For this review, take the finished solid that the model builds, in its own axes (mm). Face numbers are marked on the shaded views. A direction names the side the tool comes from. Coordinates: 2 decimals unless noted, no trailing zeros. Order: outer loops, then holes, each group sorted by start corner. A loop starts at its lowest first (then second) coordinate and runs counter-clockwise, first axis right, second up. Notation, with made-up numbers: M -1.5,-18 L 47.5,-18 A9 ccw 47.5,-9 Z; hole C -34.75,-33.75 d4. An arc over 180 degrees is marked long. Use CSV: the item, a comma, the result in double quotes.
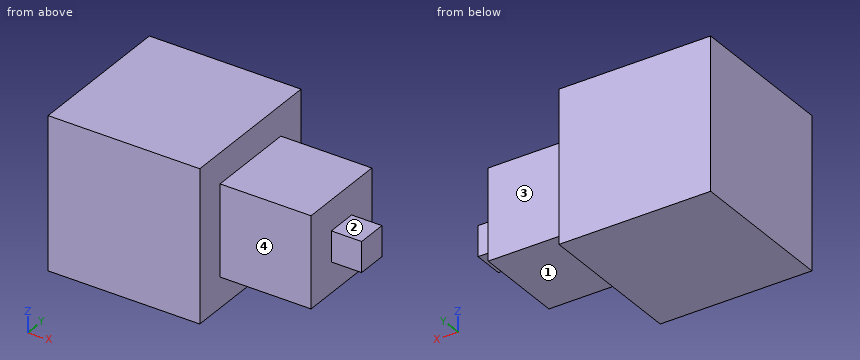
```python
from build123d import *

# Parameters (mm, degrees)
F0_W     = 100
F0_H     = 100
F1_DEPTH = 99.9998
F2_W     = 60
F2_H     = 60
F3_DEPTH = 60
F4_W     = 20
F4_H     = 20
F5_DEPTH = 20


with BuildPart() as f1:
    # F0 (on Right) → F1 (new body)
    with BuildSketch(Plane.YZ):
        with Locations((-0.458728, -3.978418)):
            Rectangle(F0_W, F0_H)
    extrude(amount=F1_DEPTH)

    # F2 (on face) → F3 (join)
    with BuildSketch(Plane.YZ.offset(99.9998)):
        with Locations((-0.458728, -3.978418)):
            Rectangle(F2_W, F2_H)
    extrude(amount=F3_DEPTH)

    # F4 (on face) → F5 (join)
    with BuildSketch(Plane.YZ.offset(159.9998)):
        with Locations((-0.458728, -3.978418)):
            Rectangle(F4_W, F4_H)
    extrude(amount=F5_DEPTH)


solid = f1.part
```
Item 1: For the marked faces 1, 2, 3 and 4, list the 3-axis set-ups (+Z, -Z, +X, -X, +Y, -Y) from which the entire face can be reached by the end or side of a thin tool; tool diameter is ignored.
Solutions:
face 1,"-Z, +X, +Y, -Y"
face 2,"+Z, +X, +Y, -Y"
face 3,"+Z, -Z, +X, +Y"
face 4,"+Z, -Z, +X, -Y"
Item 2: To check wall thickness, follow line 1 along Y through (x, z) = (134.5, -10); line 2 along X through (y, z) = (11, 28.5); line 3 along X through (y, z) = (-24, -3.5). State the ranges of each line that lie inside material, in increasing order. Write a range as [from, to].
Solutions:
line 1,"[-30.46, 29.54]"
line 2,"[0, 100]"
line 3,"[0, 160]"
Item 3: Add section B-B on z = -1. State the section outline as (x, y) points.
Solutions:
outline,"M 0,-50.46 L 100,-50.46 L 100,-30.46 L 160,-30.46 L 160,-10.46 L 180,-10.46 L 180,9.54 L 160,9.54 L 160,29.54 L 100,29.54 L 100,49.54 L 0,49.54 Z"
Item 4: Clearance check with flat-ended pins moving along their axes: pin 1 Ø5 at (y, z) = (23, -6.5) entering from -X; pin 2 Ø16 at (x, z) = (172.5, -3.5) entering from +Y; pin 3 Ø1 at (x, y) = (118, -8.5) entering from -Z; pin 4 Ø6 at (x, y) = (171, 3) entering from +Z. State where each tip first meets the part, or that it passes through.
Solutions:
pin 1,"x = 0"
pin 2,"y = 9.54"
pin 3,"z = -33.98"
pin 4,"z = 6.02"
Item 5: Add section D-D on z = -19. State the section outline as (x, y) points.
Solutions:
outline,"M 0,-50.46 L 100,-50.46 L 100,-30.46 L 160,-30.46 L 160,29.54 L 100,29.54 L 100,49.54 L 0,49.54 Z"
Item 6: Add section C-C on x = 144. State the section outline as (y, z) points, and give its area (3 significant figures).
Solutions:
outline,"M -30.46,-33.98 L 29.54,-33.98 L 29.54,26.02 L -30.46,26.02 Z"
area,"3,600 mm^2"
Item 7: Add section A-A on y = 13.5. State the section outline as (x, z) points, and give its area (3 significant figures).
Solutions:
outline,"M 0,-53.98 L 100,-53.98 L 100,-33.98 L 160,-33.98 L 160,26.02 L 100,26.02 L 100,46.02 L 0,46.02 Z"
area,"13,600 mm^2"
